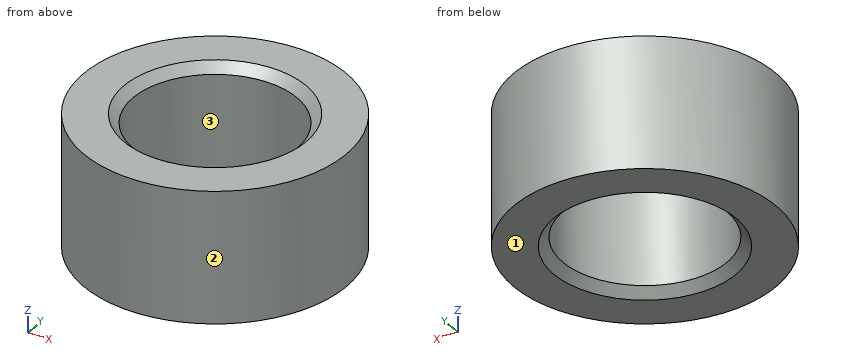
```python
from build123d import *

# Parameters (mm, degrees)
F0_R     = 7.2
F1_DEPTH = 7.2
F2_R     = 4.5
F3_DEPTH = 7.201
F4_SIZE  = 0.5


with BuildPart() as f1:
    # F0 (on Top) → F1 (new body)
    with BuildSketch(Plane.XY):
        Circle(F0_R)
    extrude(amount=F1_DEPTH)

    # F2 (on face) → F3 (cut, through all)
    with BuildSketch(Plane.XY.offset(7.2)):
        Circle(F2_R)
    extrude(amount=-F3_DEPTH, mode=Mode.SUBTRACT)

    # F4
    f4_edges = [f1.edges().sort_by_distance(p)[0] for p in [
        (-4.5, 0, 7.2),
        (-4.5, 0, 0),
    ]]
    chamfer(f4_edges, length=F4_SIZE)


solid = f1.part
```
Could you check a few things on this model? Use its own coordinates, in mm. Face numbers are marked on the shaded views. Round coordinates to 2 decimals unless told otherwise and drop trailing zeros. Loops run counter-clockwise (first coordinate to the right, second up) from the corner with the lowest first, then second, coordinate; pieces in that order, holes last.
Q1. I want a section at C-C (z = 4.5). Write out the boundary of the cut face in (x, y), and give its area (3 significant figures).
Q2. For P1, Ø8, axis at x = -3.5, y = 2.5, coming from the +Z side; P2, Ø1.5, axis at y = -5, z = 3, coming from the +X side; P3, Ø4, axis at y = 5.5, z = 1.5, coming from the -X side; P4, Ø5, axis at x = 1.5, y = 0.5, coming from the -Z side, each with a flat end and sliding along its axis, tell me the tip position at first contact or that it passes through.
Q3. I want a section at A-A (x = 0). Write out the boundary of the cut face in (y, z).
Q4. I want a section at D-D (y = 5.25). Write out the boundary of the cut face in (x, z).
Q5. Thinking about a two-plate mould opening in X: for the marked faces 1, 2 and 3, which applies, pulls with the +X half, pulls with the -X half, needs draft (parallel to the pull), parting line crosses it, or undercut?
Q6. Please list where these lines run through material, in increasing order: L1, parallel to Y at x = 0, z = 5.25; L2, parallel to X at y = -1, z = 3.5; L3, parallel to X at y = 1.25, z = 6.
Answer below:
1. outline: circle Ø14.4 at (0, 0); hole circle Ø9 at (0, 0)
1. area: 99.2 mm2
2. P1: stops at z = 7.2
2. P2: stops at x = 5.81
2. P3: stops at x = -6.29
2. P4: passes through
3. outline: (-7.2, 0) - (-5, 0) - (-4.5, 0.5) - (-4.5, 6.7) - (-5, 7.2) - (-7.2, 7.2) - close; (4.5, 0.5) - (5, 0) - (7.2, 0) - (7.2, 7.2) - (5, 7.2) - (4.5, 6.7) - close
4. outline: (-4.93, 0) - (4.93, 0) - (4.93, 7.2) - (-4.93, 7.2) - close
5. face 1: needs draft
5. face 2: parting line crosses it
5. face 3: undercut
6. L1: y = -7.2 to -4.5, 4.5 to 7.2
6. L2: x = -7.13 to -4.39, 4.39 to 7.13
6. L3: x = -7.09 to -4.32, 4.32 to 7.09
